```python
from build123d import *

# Parameters (mm, degrees)
F1_DEPTH = 50
F2_R     = 20
F3_SIZE  = 5


with BuildPart() as f1:
    # F0 (on Front) → F1 (new body)
    with BuildSketch(Plane.XZ):
        Polygon((0, -25), (25, -25), (25, 25), (0, 68.30127), (-25, 25), (-25, -25), (-5, -25), (-5, -4.773571), (0, -4.773571), align=None)
    extrude(amount=F1_DEPTH)

    # F2
    f2_edges = [f1.edges().sort_by_distance(p)[0] for p in [
        (0, -25, 68.30127),
    ]]
    fillet(f2_edges, radius=F2_R)

    # F3
    f3_edges = [f1.edges().sort_by_distance(p)[0] for p in [
        (25, 0, 0),
        (-25, 0, 0),
    ]]
    chamfer(f3_edges, length=F3_SIZE)


solid = f1.part
```
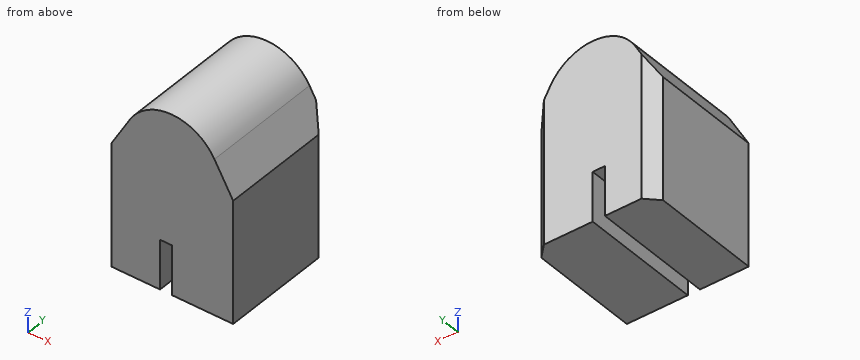
Geometry: final body of the model. Coordinates: model frame, mm. Give positions to 0.01 mm unless a question says otherwise; leave off trailing zeros. Loops run counter-clockwise (first coordinate to the right, second up) from the corner with the lowest first, then second, coordinate; pieces in that order, holes last. Notation, with made-up numbers: (66.25, 10) - (72.25, 10) arc R25 cw to (72.25, 29) - close; hole circle Ø3 at (-18.75, 83.25). An arc over 180 degrees is marked (long way). Answer as CSV lines item,"result". Start each with the question number.
(1) Section query A-A (y = -35). Output: boundary loops of the cut face in (x, z), and give its area (3 significant figures).
(2) Section query D-D (x = 7). Output: boundary loops of the cut face in (y, z).
(3) Ray query, line 1 along X through (y, z) = (-17.5, -13); line 2 along Z through (x, y) = (-17, -2.5); line 3 along X through (y, z) = (-14.5, 37.5). Return the intervals inside material, ascending. Write a range as [from, to].
(4) Section query B-B (z = 31.5). Output: boundary loops of the cut face in (x, y), and give its area (3 significant figures).
(5) Section query C-C (x = -16.5). Output: boundary loops of the cut face in (y, z).
(6) Pin query (flat end, axial travel): P1, Ø1, axis at x = 17, y = -31.5, coming from the +Z side. Return the tip coordinate at first contact, or that it passes through.
Worked answers:
1,outline,"(-25, -25) - (-5, -25) - (-5, -4.77) - (0, -4.77) - (0, -25) - (25, -25) - (25, 25) - (17.32, 38.3) arc R20 ccw to (-17.32, 38.3) - (-25, 25) - close"
1,area,"3,210 mm^2"
2,outline,"(-50, -25) - (0, -25) - (0, 47.04) - (-50, 47.04) - close"
3,line 1,"x = [-25, -5], [0, 25]"
3,line 2,"z = [-25, 38.84]"
3,line 3,"x = [-17.78, 17.78]"
4,outline,"(-21.25, -50) - (21.25, -50) - (21.25, -1.25) - (20, 0) - (-20, 0) - (-21.25, -1.25) - close"
4,area,"2,120 mm^2"
5,outline,"(-50, -25) - (0, -25) - (0, 39.6) - (-50, 39.6) - close"
6,P1,"stops at z = 39.6"
